Geometry: final body of the model. Coordinates: model frame, mm. Face numbers are marked on the shaded views. A direction names the side the tool comes from. Give positions to 0.01 mm unless a question says otherwise; leave off trailing zeros. Answer in a Markdown table with one row per item.
Autodesk Inventor part; units mm, degrees
ref_plane "Top Plane" through (-7.3, 8.6, -7.3) normal (0, 1, 0) x (1, 0, 0)
ref_plane "YZ Plane" through (0, 0, 0) normal (1, 0, 0) x (0, 1, 0)
ref_plane "XZ Plane" through (0, 0, 0) normal (0, 1, 0) x (-1, 0, 0)
sketch "Base Loop" plane through (0, 0, 0) normal (0, 1, 0) x (-1, 0, 0)
  line L0 (-7.3, 7.3) -> (7.3, 7.3)
  line L1 (7.3, 7.3) -> (7.3, -7.3)
  line L2 (7.3, -7.3) -> (-7.3, -7.3)
  line L3 (-7.3, -7.3) -> (-7.3, 7.3)
  line L4 (-7.3, 7.3) -> (7.3, -7.3) construction
  line L5 (7.3, 7.3) -> (-7.3, -7.3) construction
  point P0 (0, 0)
  point P1 (0, 0)
  point P2 (0, 0)
  dimension "d0" = 14.6
  dimension "d1" = 14.6
ref_plane "Mid Plane" through (-7.3, 2, -7.3) normal (0, 1, 0) x (1, 0, 0)
ref_plane "Base Plane" through (-7.3, 0, -7.3) normal (0, 1, 0) x (1, 0, 0)
sketch "Mid Loop" plane through (-7.3, 2, -7.3) normal (0, 1, 0) x (1, 0, 0)
  line L0 (14.5, -14.5) -> (0.1, -14.5)
  line L1 (0.1, -14.5) -> (0.1, -0.1)
  line L2 (0.1, -0.1) -> (14.5, -0.1)
  line L3 (14.5, -0.1) -> (14.5, -14.5)
  line L4 (14.5, -14.5) -> (0.1, -0.1) construction
  line L5 (0.1, -14.5) -> (14.5, -0.1) construction
  point P0 (7.3, -7.3)
  dimension "d3" = 14.4
  dimension "d4" = 14.4
ref_plane "Top Plane" through (-7.3, 8.6, -7.3) normal (0, 1, 0) x (1, 0, 0)
sketch "Top Loop" plane through (-7.3, 8.6, -7.3) normal (0, 1, 0) x (1, 0, 0)
  line L0 (13.3, -13.3) -> (1.3, -13.3)
  line L1 (1.3, -13.3) -> (1.3, -1.3)
  line L2 (1.3, -1.3) -> (13.3, -1.3)
  line L3 (13.3, -1.3) -> (13.3, -13.3)
  line L4 (13.3, -13.3) -> (1.3, -1.3) construction
  line L5 (1.3, -13.3) -> (13.3, -1.3) construction
  point P0 (7.3, -7.3)
  dimension "d6" = 12
  dimension "d7" = 12
loft "Keyswitch Body" add profiles "Base Loop", "Mid Loop", "Top Loop"
sketch "Cut in profile" plane through (-6, 8.6, 6) normal (0, 1, 0) x (1, 0, 0)
  line L0 (8.7, 2.275) -> (3.3, 2.275)
  line L1 (3.3, 2.275) -> (3.3, 9.725)
  line L2 (3.3, 9.725) -> (8.7, 9.725)
  line L3 (8.7, 9.725) -> (8.7, 2.275)
  line L4 (8.7, 2.275) -> (3.3, 9.725) construction
  line L5 (3.3, 2.275) -> (8.7, 9.725) construction
  point P0 (6, 6)
  dimension "d17" = 7.45
  dimension "d18" = 5.4
extrude "Pole Cut in" cut sketch "Cut in profile" against normal blind 6.6
equation "\"d1\" = d0"
equation "\"d3\" = s_bwidth"
equation "\"d4\" = d3"
equation "\"d17\" = s_polebl"
equation "\"d18\" = s_polebw"
equation "\"k_width\" = 18"
equation "\"k_height\" = 16.5"
equation "\"k_taper1\" = 1.5"
equation "\"k_taper2\" = 0.5"
equation "\"k_radius\" = 6"
equation "\"k_wthick\" = 1.5"
equation "\"k_ribthick\" = 1.5"
equation "\"k_ribheight\" = 5"
equation "\"k_poleoff\" = 2.25"
equation "\"k_poledia\" = 5.3"
equation "\"k_cmxw\" = 1.1"
equation "\"k_cmxl\" = 4.15"
equation "\"s_bwidth\" = 14.4"
equation "\"s_poleh\" = 3.6"
equation "\"s_polebw\" = 5.4"
equation "\"s_polebl\" = 7.45"
equation "\"b_rshift\" = 49.5"
equation "\"b_ctrl\" = 22.5"
equation "\"b_space\" = 117"
equation "\"b_height\" = 77"
equation "\"b_width\" = 285"
equation "\"b_lshift\" = 40.5"
equation "\"b_tab\" = 27"
equation "\"b_pad\" = 1"
equation "\"b_caps\" = 31.5"
equation "\"k_staper\" = 1"
equation "\"k_ltaper\" = 1.5"
equation "\"k_lradius\" = 6"
equation "\"k_sradius\" = 4"
equation "\"k_height_t\" = 16"
equation "\"k_taper_wide\" = 1.5"
equation "\"k_taper_thin\" = 0.0001"
equation "\"k_height_low\" = 15"
equation "\"k_shortening\" = 4.5"
equation "\"k_cmxd\" = 4"
equation "\"k_taper_side\" = 0.5"
properties part number "keyswitch-base_cherrymx"
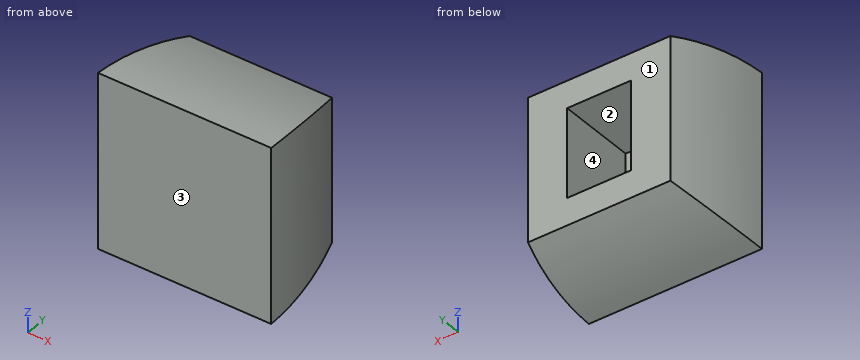
Q1. Material intervals for line 1 along Y through (x, z) = (-0.25, 0); line 2 along X through (y, z) = (2.5, 3.5); line 3 along X through (y, z) = (5, -3.25), sorted ascending.
Check values:
| item | result |
|---|---|
| line 1 | 0 to 2 |
| line 2 | -7.16 to -2.7, 2.7 to 7.16 |
| line 3 | -6.83 to -2.7, 2.7 to 6.83 |
Q2. Reachability of the marked faces 1 and 2 from +Z, -Z, +X, -X, +Y, -Y: full face, straight path, thin tool, end or side. Return the list, or none.
Check values:
| item | result |
|---|---|
| face 1 | +Z, -Z, +X, -X, +Y |
| face 2 | +Y |
Q3. Draft query along Z for the marked faces 3 and 4. Return one class per face: pulls with the +Z half, pulls with the -Z half, needs draft (parallel to the pull), parting line crosses it, or undercut.
Check values:
| item | result |
|---|---|
| face 3 | needs draft |
| face 4 | undercut |
Q4. First-contact query: pin 1 (4.5 mm diameter, centred on x = 1.5, y = 4, fed in from +Z); pin 2 (3 mm diameter, centred on x = -3, y = 2.5, fed in from -Z); pin 3 (3.5 mm diameter, centred on y = 6.5, z = 1.5, fed in from -X). Flat tips, straight axial feed; report the tip coordinate or a pass-through.
Check values:
| item | result |
|---|---|
| pin 1 | z = 7.22 |
| pin 2 | z = -7.26 |
| pin 3 | x = -6.87 |
